Input: part model. Units: mm. Frame: model coordinates. A direction names the side the tool comes from. Round coordinates to 2 decimals unless told otherwise and drop trailing zeros. Loops run counter-clockwise (first coordinate to the right, second up) from the corner with the lowest first, then second, coordinate; pieces in that order, holes last. Notation, with made-up numbers: M 36,60.25 L 83,60.25 A15 ccw 83,65.25 Z; hole C -16,34.25 d5. An arc over 180 degrees is marked long. Put each result on its own line as item: value. Start each with the question number.
1) Section A-A on y = 18. Output: boundary loops of the cut face in (x, z), plus the area to 3 significant figures.
2) Pin query (flat end, axial travel): pin 1 (4 mm diameter, centred on y = 105.5, z = -5.5, fed in from +X); pin 2 (4 mm diameter, centred on x = -9, y = 60.5, fed in from +Z); pin 3 (4 mm diameter, centred on x = 2.5, y = 85, fed in from -Z); pin 4 (18.5 mm diameter, centred on x = 0.5, z = -15, fed in from -Y). Return the tip coordinate at first contact, or that it passes through.
3) Line query: probe 1 along X at (y, z) = (27, 0); probe 2 along X at (y, z) = (115.75, 0). Output: solid intervals per line, ascending.
4) Draft query along X for faces 1 (the face through (-30.736, 68.374, 4.036)), 2 (the face through (20.5, 77.1, -22.8)), 3 (the face through (20.074, 111.404, 4.458)). Return one class per face: +X half, -X half, draft (parallel to the pull), parting line (faces both ways), or undercut.
5) Reachability of faces 4 (the face through (-30.736, 49.425, 4.036)), 5 (the face through (0, 2, 0)) from +Z, -Z, +X, -X, +Y, -Y: full face, straight path, thin tool, end or side. Return the list, or none.
from build123d import *


with BuildPart() as part:
    # Sketch1 → Bottle_body_revolve (revolve)
    with BuildSketch(Plane.XY, mode=Mode.PRIVATE) as bottle_body_revolve_sk:
        Polygon((0, 0), (29, 0), (31, 2), (31, 20.3), (30.4, 20.3), (30.4, 21.5), (31, 21.5), (31, 39.2), (30.4, 39.2), (30.4, 40.4), (31, 40.4), (31, 58.2), (30.4, 58.2), (30.4, 59.4), (31, 59.4), (31, 77.1), (30.4, 77.1), (30.4, 78.3), (31, 78.3), (31, 95), (22, 113), (22, 125), (20, 125), (20, 112.53), (29, 94.53), (29, 2), (0, 2), align=None)
    revolve(bottle_body_revolve_sk.sketch.rotate(Axis((0, -10, 0), (0, 1, 0)), 90), axis=Axis((0, -10, 0), (0, 1, 0)))


solid = part.part
Geometry results:
1. outline: C 0,0 d62; hole C 0,0 d58
1. area: 377 mm²
2. pin 1: stops at x = 26.25
2. pin 2: stops at z = 30.2
2. pin 3: stops at z = -31
2. pin 4: stops at y = 0
3. probe 1: x = -31 to -29, 29 to 31
3. probe 2: x = -22 to -20, 20 to 22
4. face 1: parting line
4. face 2: draft
4. face 3: undercut
5. face 4: +Y, -Y
5. face 5: none
